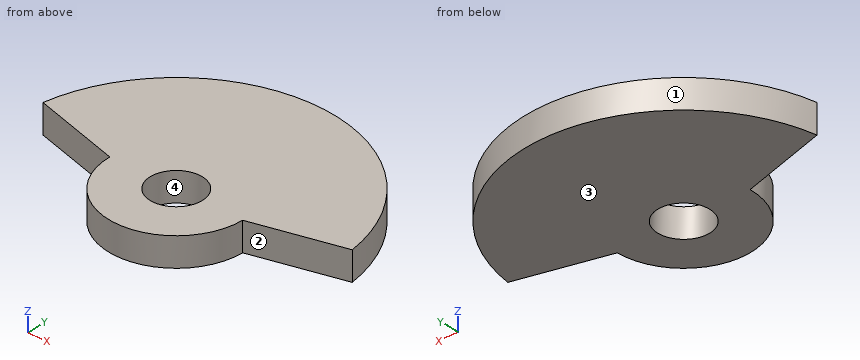
from build123d import *

# Parameters (mm, degrees)
SZKIC1_R                    = 9
DODANIE_WYCI_GNI_CIE1_DEPTH = 10


with BuildPart() as part:
    # Szkic1 → Dodanie-wyciągnięcie1 (new body)
    with BuildSketch(Plane.XY):
        with BuildLine():
            Line((-23.35, 0), (-54.368386356, 8.311351575))
            ThreePointArc((-54.368386356, 8.311351575), (0, 55), (54.368386356, 8.311351575))
            Line((54.368386356, 8.311351575), (23.35, 0))
            ThreePointArc((23.35, 0), (0, -23.35), (-23.35, 0))
        make_face()
        Circle(SZKIC1_R, mode=Mode.SUBTRACT)
    extrude(amount=DODANIE_WYCI_GNI_CIE1_DEPTH)


solid = part.part
Source: CAD feature listing. Evaluate the final solid. Frame: model axes, mm. Face numbers are marked on the shaded views. Give positions to 0.01 mm unless a question says otherwise; leave off trailing zeros. Write each loop counter-clockwise with the first axis right and the second up, starting at its lowest first coordinate (ties: lowest second). Pieces come first, ordered by that corner, then holes. Notation, with made-up numbers: M 5.5,7 L 31.5,7 A30 ccw 31.5,30 Z; hole C 44,-10.5 d1. An arc over 180 degrees is marked long. Return JSON: item names as keys, results as strings. Group by question number.
1) Cut plane C-C, the plane z = 8. Output: boundary loops of the cut face in (x, y).
2) Pin query (flat end, axial travel): P1, Ø6, axis at x = -26.5, z = 4, coming from the -Y side; P2, Ø6, axis at y = 16, z = 3.5, coming from the +X side; P3, Ø2, axis at x = -40.5, z = 1.5, coming from the -Y side; P4, Ø16, axis at x = 0, y = 0, coming from the -Z side. Return the tip coordinate at first contact, or that it passes through.
3) Cut plane A-A, the plane x = 0. Output: boundary loops of the cut face in (y, z).
4) Pull-direction query (Y, two-part tool) for the marked faces 1, 2, 3 and 4; classes: pulls with the +Y half, pulls with the -Y half, needs draft (parallel to the pull), parting line crosses it, or undercut.
5) Material intervals for line 1 along Y through (x, z) = (0, 2); line 2 along Y through (x, z) = (2.5, 0.75); line 3 along Y through (x, z) = (-24, 0.5), sorted ascending. Write a range as [from, to].
6) Cut plane D-D, the plane y = -14.5. Output: boundary loops of the cut face in (x, z).
7) Cut plane B-B, the plane y = -4.5. Output: boundary loops of the cut face in (x, z), plus the area to 3 significant figures.
Recorded:
{
 "1": {"outline": "M -54.37,8.31 L -23.35,0 A23.35 ccw 23.35,0 L 54.37,8.31 A55 ccw Z; hole C 0,0 d18"},
 "2": {"P1": "stops at y = 0.04", "P2": "stops at x = 53.44", "P3": "stops at y = 4.33", "P4": "passes through"},
 "3": {"outline": "M -23.35,0 L -9,0 L -9,10 L -23.35,10 Z; M 9,0 L 55,0 L 55,10 L 9,10 Z"},
 "4": {"face 1": "pulls with the +Y half", "face 2": "pulls with the -Y half", "face 3": "needs draft", "face 4": "undercut"},
 "5": {"line 1": "y = [-23.35, -9], [9, 55]", "line 2": "y = [-23.22, -8.65], [8.65, 54.94]", "line 3": "y = [0.17, 49.49]"},
 "6": {"outline": "M -18.3,0 L 18.3,0 L 18.3,10 L -18.3,10 Z"},
 "7": {"outline": "M -22.91,0 L -7.79,0 L -7.79,10 L -22.91,10 Z; M 7.79,0 L 22.91,0 L 22.91,10 L 7.79,10 Z", "area": "302 mm²"}
}
